For this review, take the finished solid that the model builds, in its own axes (mm). Face numbers are marked on the shaded views. A direction names the side the tool comes from. Coordinates: 2 decimals unless noted, no trailing zeros. Loops run counter-clockwise (first coordinate to the right, second up) from the corner with the lowest first, then second, coordinate; pieces in that order, holes last.
1. Take a section at C-C, the plane z = 0. Count the separate pieces of the cut face and the enclosed holes in it, then the cut area to 3 significant figures.
2. Take a section at D-D, the plane x = 11.5. State the section outline as (y, z) points (3 decimals).
3. Mouldability with a two-part tool opening along X and no side actions: class the marked faces 1, 2, 3 and 4 as pulls with the +X half, pulls with the -X half, needs draft (parallel to the pull), parting line crosses it, or undercut.
4. Take a section at B-B, the plane z = 4.75. State the section outline as (x, y) points (3 decimals).
5. To check wall thickness, follow probe 1 along X at (y, z) = (4.5, 4) (3 decimals); probe 2 along X at (y, z) = (0.6, 0); probe 3 along X at (y, z) = (5.75, -1) (3 decimals). State the ranges of each line that lie inside material, in increasing order.
6. Clearance check with flat-ended pins moving along their axes: P1, Ø1, axis at y = 6.5, z = 0.5, coming from the -X side (3 decimals); P2, Ø6, axis at x = 22.5, z = 1.5, coming from the -Y side; P3, Ø1, axis at x = 8, z = 0.5, coming from the +Y side (3 decimals). State where each tip first meets the part, or that it passes through.
7. Take a section at A-A, the plane x = 15. State the section outline as (y, z) points (3 decimals).
8. Machinability: for the marked faces 5, 6 and 7, which of the approach directions +Z, -Z, +X, -X, +Y, -Y give a long, thin tool a straight path to every point of the face, cutting with its end or side? Answer none if there is none.
```python
from build123d import *

# Parameters (mm, degrees)
SKETCH1_R           = 2.286
BOSS_EXTRUDE1_DEPTH = 3.175
SKETCH5_W           = 3.175
SKETCH5_H           = 10.922
BOSS_EXTRUDE5_DEPTH = 2.54
BOSS_EXTRUDE6_START = 9.525
BOSS_EXTRUDE6_DEPTH = 3.175
BOSS_EXTRUDE7_DEPTH = 13.97
SKETCH10_R          = 3.1115
CUT_EXTRUDE1_DEPTH  = 3.175
CHAMFER1_SIZE       = 2.54
CHAMFER1_SIZE2      = 3.592102448


# Read off the part's stored shape, not the designer's step: Boss-Extrude6
with BuildPart() as part:
    # Sketch1 → Boss-Extrude1 (new body)
    with BuildSketch(Plane(origin=(0, 0, 0), x_dir=(1, 0, 0), z_dir=(0, 1, 0))):
        with BuildLine():
            Line((0, 5.461), (12.7, 5.461))
            Line((12.7, 5.461), (12.7, -5.461))
            Line((12.7, -5.461), (0, -5.461))
            ThreePointArc((0, -5.461), (-5.461, 0), (0, 5.461))
        make_face()
        with Locations(Location((0, 0, 0), (0, 0, 270))):
            Circle(SKETCH1_R, mode=Mode.SUBTRACT)
    extrude(amount=BOSS_EXTRUDE1_DEPTH)

    # Sketch5 → Boss-Extrude5 (add)
    with BuildSketch(Plane(origin=(0, 3.175, 0), x_dir=(1, 0, 0), z_dir=(0, 1, 0))):
        with Locations((11.1125, 0)):
            Rectangle(SKETCH5_W, SKETCH5_H)
    extrude(amount=BOSS_EXTRUDE5_DEPTH)

    # Boss-Extrude6 outline → Boss-Extrude6 (add)
    with BuildSketch(Plane.YZ.offset(BOSS_EXTRUDE6_START)):
        Polygon((16.637, 5.461), (5.715, 5.461), (5.715, -5.461), align=None)
    extrude(amount=BOSS_EXTRUDE6_DEPTH)

    # Sketch9 → Boss-Extrude7 (add)
    with BuildSketch(Plane(origin=(12.7, 0, 0), x_dir=(0, 0, -1), z_dir=(1, 0, 0))):
        Polygon((-5.461, 16.637), (-5.461, 12.146871939), (2.921, 3.764871939), (2.921, 0), (5.461, 0), (5.461, 1.224871939), (5.461, 5.715), align=None)
    extrude(amount=BOSS_EXTRUDE7_DEPTH)

    # Sketch10 → Cut-Extrude1 (cut)
    with BuildSketch(Plane(origin=(0, 5.588, -5.588), x_dir=(1, 0, 0), z_dir=(0, 0.7071067811865465, -0.7071067811865487))):
        with Locations(Location((20.32, -6.529605122, 0), (0, 0, 270))):
            Circle(SKETCH10_R)
    extrude(amount=-CUT_EXTRUDE1_DEPTH, mode=Mode.SUBTRACT)

    # Chamfer1
    chamfer1_edges = [part.edges().sort_by_distance(p)[0] for p in [
        (18.0975, 16.637, 5.461),
    ]]
    chamfer1_side = [part.faces().sort_by_distance(p)[0] for p in [
        (12.385662813, 6.07343597, 5.461),
    ]]
    chamfer(chamfer1_edges, length=CHAMFER1_SIZE, length2=CHAMFER1_SIZE2, reference=chamfer1_side[0])


solid = part.part
```
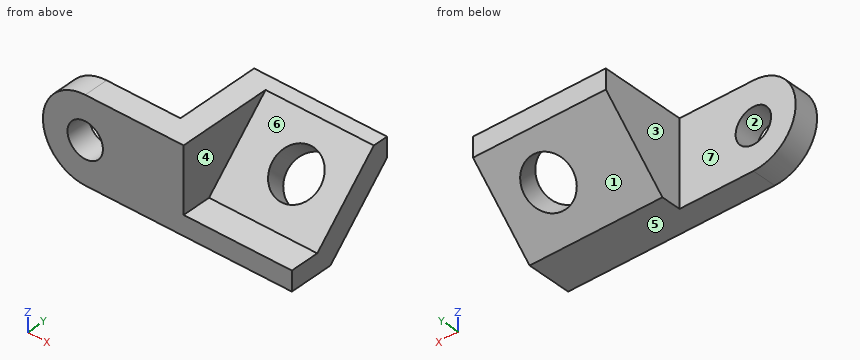
Results list:
1. separate pieces: 3
1. enclosed holes: 0
1. area: 105 mm2
2. outline: (0, -5.461) - (5.715, -5.461) - (14.097, 2.921) - (14.097, 5.461) - (0, 5.461) - close
3. face 1: needs draft
3. face 2: undercut
3. face 3: pulls with the -X half
3. face 4: pulls with the +X half
4. outline: (-2.694, 0) - (12.7, 0) - (12.7, 11.436) - (26.67, 11.436) - (26.67, 14.097) - (9.525, 14.097) - (9.525, 3.175) - (-2.694, 3.175) - close
5. probe 1: x = 9.525 to 12.7
5. probe 2: x = -5.46 to -2.29, 2.29 to 12.7
5. probe 3: x = 9.525 to 26.67
6. P1: stops at x = 9.525
6. P2: stops at y = 5.19
6. P3: stops at y = 3.175
7. outline: (0, -5.461) - (5.715, -5.461) - (14.097, 2.921) - (14.097, 5.461) - (12.147, 5.461) - (3.765, -2.921) - (0, -2.921) - close
8. face 5: -Z, +X, -X, +Y, -Y
8. face 6: +Z, +X, -Y
8. face 7: +Z, -Z, -X, +Y
